The model under review builds one solid part; all positions refer to its coordinate system, in mm. Give positions to 0.01 mm unless a question says otherwise; leave off trailing zeros. Loops run counter-clockwise (first coordinate to the right, second up) from the corner with the lowest first, then second, coordinate; pieces in that order, holes last. Notation, with made-up numbers: (16, 35.25) - (27, 35.25) arc R18 cw to (27, 49.25) - close; hole circle Ø2 at (-31.75, 45.5). An arc over 180 degrees is marked (long way). Return JSON: item names as keys, results as strings. Group by question number.
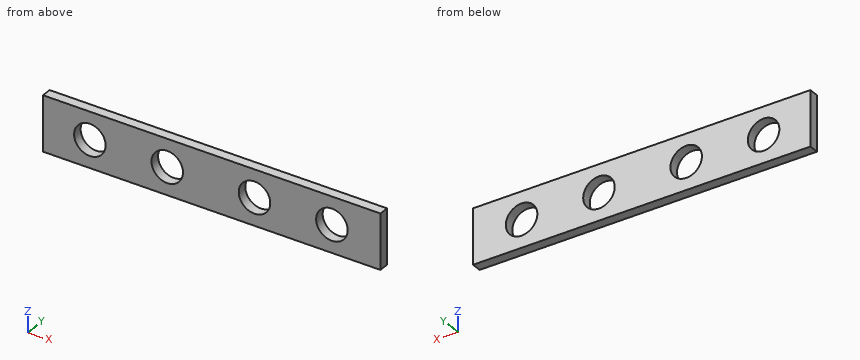
Autodesk Inventor part; units mm, degrees
ref_plane "YZ Plane" through (0, 0, 0) normal (1, 0, 0) x (0, 1, 0)
ref_plane "XZ Plane" through (0, 0, 0) normal (0, 1, 0) x (-1, 0, 0)
ref_plane "XY Plane" through (0, 0, 0) normal (0, 0, 1) x (1, 0, 0)
sketch "Sketch1" plane through (0, 0, 0) normal (0, 1, 0) x (-1, 0, 0)
  line L0 (0, 0) -> (0, -14)
  line L1 (0, -14) -> (85.598, -14)
  line L2 (85.598, -14) -> (85.598, 0)
  line L3 (85.598, 0) -> (0, 0)
  dimension "d0" = 14
  dimension "d1" = 85.598
extrude "Extrusion1" add sketch "Sketch1" along normal blind 2.5
sketch "Sketch2" plane through (0, 2.5, 0) normal (0, 1, 0) x (1, 0, 0)
  line L0 (0, 0) -> (0, 14)
  line L1 (0, 14) -> (-85.598, 14)
  line L2 (-85.598, 0) -> (0, 0)
  circle A0 centre (-12.3165, 7) radius 4
  circle A1 centre (-31.949, 7) radius 4
  line L3 (0, 0) -> (-85.598, 0)
  line L4 (0, 24) -> (-2.5, 24)
  line L5 (-2.5, 24) -> (-41.766, 24)
  line L6 (-41.766, 24) -> (-44.266, 24)
  line L7 (-44.266, 24) -> (-54.083, 24)
  line L8 (-44.266, 24) -> (-83.532, 24)
  line L9 (-83.532, 24) -> (-73.715, 24)
  line L10 (-73.715, 24) -> (-73.715, -12)
  line L11 (-44.266, 24) -> (-44.266, -7)
  line L12 (-54.083, 24) -> (-54.083, -7)
  circle A2 centre (-54.083, 7) radius 4
  circle A3 centre (-73.715, 7) radius 4
  line L13 (-73.715, 7) -> (-12.3165, 7)
  dimension "d15" = 8
  dimension "d17" = 2.5
  dimension "d18" = 39.266
  dimension "d19" = 9.8165
  dimension "d20" = 9.817
  dimension "d21" = 2.5
  dimension "d22" = 9.817
  dimension "d23" = 39.266
  dimension "d24" = 9.817
  dimension "d25" = 8
  dimension "d27" = 8
extrude "Extrusion2" cut sketch "Sketch2" against normal blind 2.5 contours A0 | A1 L13 | L13 A1 | A2 L13 L12 | L12 L13 A2 | L13 L12 A2 | L12 L13 A2 | A3 L10 | L10 L13 A3 | A3 L13 L10
properties part number "Estructura Anillos" material "MDF Medium Density Fiberboard"
Item 1: For P1, Ø3, axis at x = -73, z = -6.5, coming from the +Y side, flat-tipped, find the tip position at first contact; note if it passes through.
Item 2: Take a section at A-A (y = 0.9). State the section outline as (x, z) points (1 decimal).
Item 3: Take a section at B-B (x = -75). State the section outline as (y, z) points.
Item 4: Take a section at C-C (z = -7). State the section outline as (x, y) points (1 decimal), then the cut area to 3 significant figures.
Item 5: Take a section at D-D (x = -12). State the section outline as (y, z) points, then the cut area to 3 significant figures.
Item 6: For L1, parallel to X at y = 1.2, z = -7 (1 decimal); L2, parallel to X at y = 0.8, z = -8.75; L3, parallel to Z at x = -72.5, y = 1.3, list the stretches that pass through material, from the lowest coordinate up. Write a range as from..to.
Check sheet entries:
{
 "1": {"P1": "passes through"},
 "2": {"outline": "(-85.6, -14) - (0, -14) - (0, 0) - (-85.6, 0) - close; hole circle Ø8 at (-73.7, -7); hole circle Ø8 at (-54.1, -7); hole circle Ø8 at (-31.9, -7); hole circle Ø8 at (-12.3, -7)"},
 "3": {"outline": "(0, -14) - (2.5, -14) - (2.5, -10.79) - (0, -10.79) - close; (0, -3.21) - (2.5, -3.21) - (2.5, 0) - (0, 0) - close"},
 "4": {"outline": "(-85.6, 0) - (-77.7, 0) - (-77.7, 2.5) - (-85.6, 2.5) - close; (-69.7, 0) - (-58.1, 0) - (-58.1, 2.5) - (-69.7, 2.5) - close; (-50.1, 0) - (-35.9, 0) - (-35.9, 2.5) - (-50.1, 2.5) - close; (-27.9, 0) - (-16.3, 0) - (-16.3, 2.5) - (-27.9, 2.5) - close; (-8.3, 0) - (0, 0) - (0, 2.5) - (-8.3, 2.5) - close", "area": "134 mm^2"},
 "5": {"outline": "(0, -14) - (2.5, -14) - (2.5, -10.99) - (0, -10.99) - close; (0, -3.01) - (2.5, -3.01) - (2.5, 0) - (0, 0) - close", "area": "15.1 mm^2"},
 "6": {"L1": "x = -85.6..-77.7, -69.7..-58.1, -50.1..-35.9, -27.9..-16.3, -8.3..0", "L2": "x = -85.6..-77.31, -70.12..-57.68, -50.49..-35.55, -28.35..-15.91, -8.72..0", "L3": "z = -14..-10.81, -3.19..0"}
}
